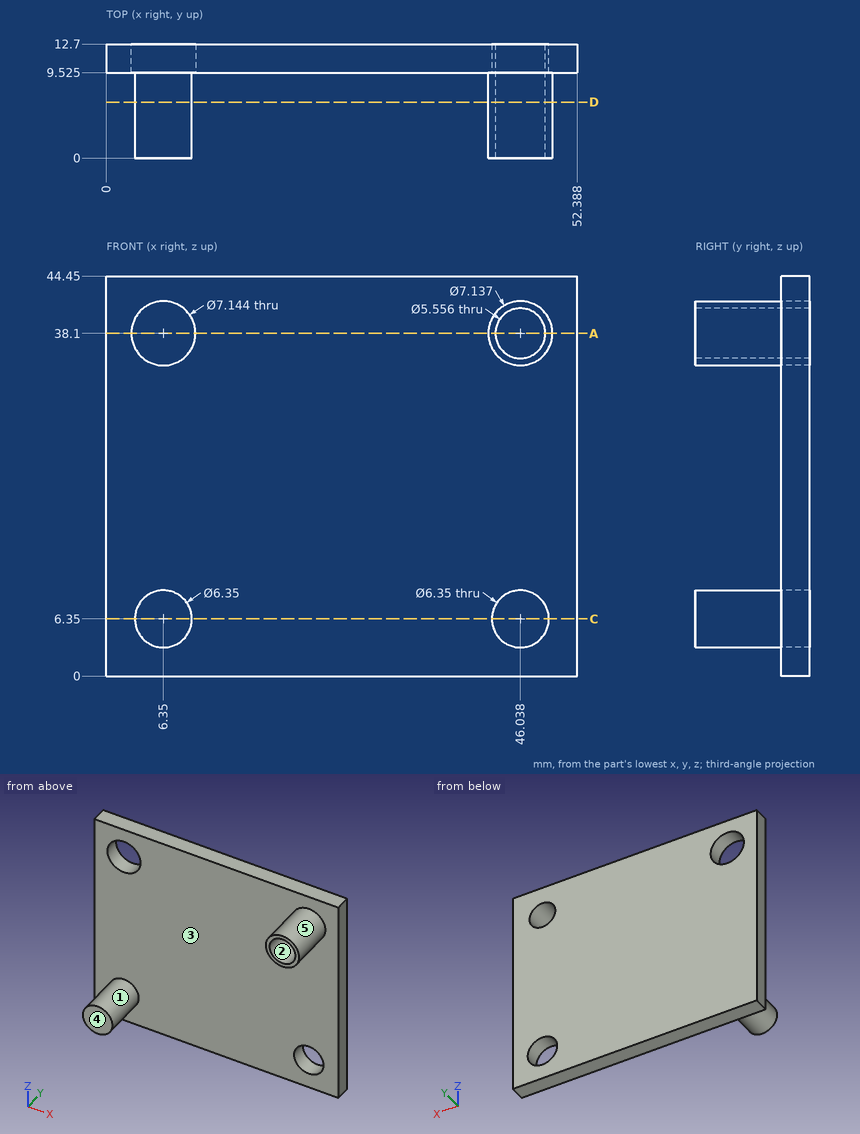
Job drawing, mm, ordinate dimensions from the low corner. One solid piece. A direction names the side the tool comes from. Give positions to 0.01 mm unless a question says otherwise; leave off trailing zeros. Order: outer loops, then holes, each group sorted by start corner. A loop starts at its lowest first (then second) coordinate and runs counter-clockwise, first axis right, second up. Notation, with made-up numbers: (83.25, 80.5) -> (134.25, 80.5) arc R14 ccw to (134.25, 98.5) -> close; hole circle Ø3 at (4, 44). An arc over 180 degrees is marked (long way). Return JSON: item names as keys, results as strings.
Q1. Saw through at A-A (z = 38.1). Write the cut outline in (x, y) (1 decimal), then the cut area to 3 significant figures.
Working result:
{"outline": "(0, 9.5) -> (2.8, 9.5) -> (2.8, 12.7) -> (0, 12.7) -> close; (9.9, 9.5) -> (42.5, 9.5) -> (42.5, 0) -> (43.3, 0) -> (43.3, 12.7) -> (9.9, 12.7) -> close; (48.8, 0) -> (49.6, 0) -> (49.6, 9.5) -> (52.4, 9.5) -> (52.4, 12.7) -> (48.8, 12.7) -> close", "area": "141 mm²"}
Q2. Saw through at D-D (y = 6.25). Count the separate pieces of the cut face and the enclosed holes in it.
Working result:
{"separate pieces": "2", "enclosed holes": "1"}
Q3. Saw through at C-C (z = 6.35). Write the cut outline in (x, y) (1 decimal), then the cut area to 3 significant figures.
Working result:
{"outline": "(0, 9.5) -> (3.2, 9.5) -> (3.2, 0) -> (9.5, 0) -> (9.5, 9.5) -> (42.9, 9.5) -> (42.9, 12.7) -> (0, 12.7) -> close; (49.2, 9.5) -> (52.4, 9.5) -> (52.4, 12.7) -> (49.2, 12.7) -> close", "area": "207 mm²"}
Q4. Drill centre lines: line 1 (Y direction, x = 4, z = 21.5) (1 decimal); line 2 (Z direction, x = 48, y = 4.5) (1 decimal); line 3 (X direction, y = 1.25, z = 9) (1 decimal). Where is each one in solid material? Low to high.
Working result:
{"line 1": "9.5 to 12.7", "line 2": "35.1 to 36.1, 40.1 to 41.1", "line 3": "4.6 to 8.1"}
Q5. Which spindle directions (+Z, -Z, +X, -X, +Y, -Y) get a long thin tool onto all of the face, cutting with end or side? Do the marked faces 4 and 5. Say none if no direction does.
Working result:
{"face 4": "+Z, -Z, +X, -X, -Y", "face 5": "-Y"}
Q6. Mould opens along Z. For the marked faces 1, 2 and 3 say: pulls with the +Z half, pulls with the -Z half, needs draft (parallel to the pull), parting line crosses it, or undercut.
Working result:
{"face 1": "parting line crosses it", "face 2": "undercut", "face 3": "needs draft"}
Q7. Flat gauge pins, fed straight in: pin 1 (5 mm diameter, centred on y = 5.5, z = 5, fed in from +X) (1 decimal); pin 2 (1 mm diameter, centred on x = 8.5, y = 4.5, fed in from -Z); pin 3 (10 mm diameter, centred on x = 46.04, z = 6.35, fed in from -Y) (1 decimal). Where does each tip first touch, or does it go through?
Working result:
{"pin 1": "x = 9.5", "pin 2": "z = 3.64", "pin 3": "y = 9.5"}
